The figure shows three views and two pictorial views of one solid part (mm, origin at its lowest corner). Answer the questions. A direction names the side the tool comes from. Coordinates: 2 decimals unless noted, no trailing zeros. Loops run counter-clockwise (first coordinate to the right, second up) from the corner with the lowest first, then second, coordinate; pieces in that order, holes last. Notation, with made-up numbers: (8, -10) - (42, -10) arc R19 cw to (42, 17) - close; hole circle Ø11 at (-32, 79.5). An arc over 180 degrees is marked (long way). Return JSON: item names as keys, results as strings. Group by question number.
1. Which of the six approach directions +Z, -Z, +X, -X, +Y, -Y give full straight-line access (tool end or side, diameter ignored) to the marked faces 1, 2, 3, 4 and 5?
2. Section A-A (x = 1.5) is taken. Write down the section's boundary in (y, z).
3. Section D-D (y = 16.5) is taken. Write down the section's boundary in (x, z).
4. Section C-C (z = 2) is taken. Write down the section's boundary in (x, y).
5. Section B-B (z = 4) is taken. Write down the section's boundary in (x, y).
6. Find the intervals of material crossed by line 1 along X through (y, z) = (5.45, 4); line 2 along Z through (x, y) = (25.5, 5.35); line 3 along Y through (x, z) = (2, 5.25), in increasing order.
7. Each of these flat-tipped pins is pushed along its axis until it touches: P1, Ø2.5, axis at x = 25.5, z = 4, coming from the +Y side; P2, Ø2.5, axis at y = 2, z = 3, coming from the -X side; P3, Ø4, axis at y = 11.5, z = 6.5, coming from the +X side. Where does it stop, or does it pass through?
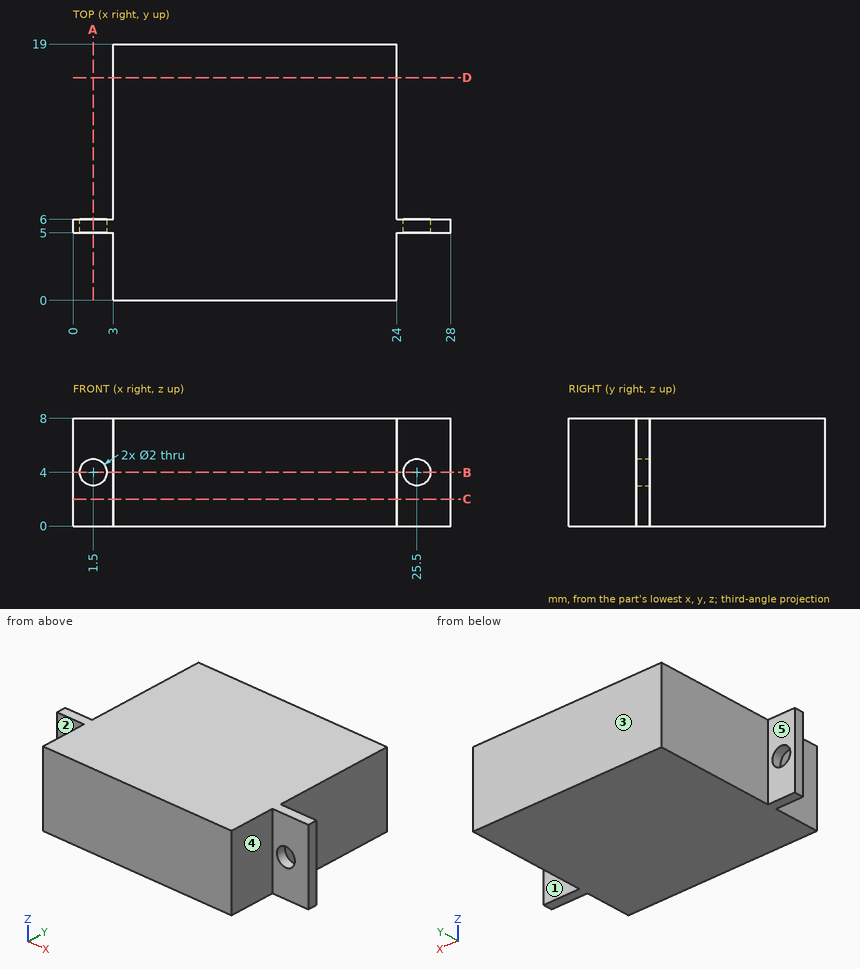
The answers:
{
 "1": {"face 1": "+Z, -Z, +X, +Y", "face 2": "+Z, -Z, -X, -Y", "face 3": "+Z, -Z, +X, -X, +Y", "face 4": "+Z, -Z, +X, -Y", "face 5": "+Z, -Z, -X, +Y"},
 "2": {"outline": "(5, 0) - (6, 0) - (6, 3) - (5, 3) - close; (5, 5) - (6, 5) - (6, 8) - (5, 8) - close"},
 "3": {"outline": "(3, 0) - (24, 0) - (24, 8) - (3, 8) - close"},
 "4": {"outline": "(0, 5) - (3, 5) - (3, 0) - (24, 0) - (24, 5) - (28, 5) - (28, 6) - (24, 6) - (24, 19) - (3, 19) - (3, 6) - (0, 6) - close"},
 "5": {"outline": "(0, 5) - (0.5, 5) - (0.5, 6) - (0, 6) - close; (2.5, 5) - (3, 5) - (3, 0) - (24, 0) - (24, 5) - (24.5, 5) - (24.5, 6) - (24, 6) - (24, 19) - (3, 19) - (3, 6) - (2.5, 6) - close; (26.5, 5) - (28, 5) - (28, 6) - (26.5, 6) - close"},
 "6": {"line 1": "x = 0 to 0.5, 2.5 to 24.5, 26.5 to 28", "line 2": "z = 0 to 3, 5 to 8", "line 3": "y = 5 to 6"},
 "7": {"P1": "stops at y = 6", "P2": "stops at x = 3", "P3": "stops at x = 24"}
}
